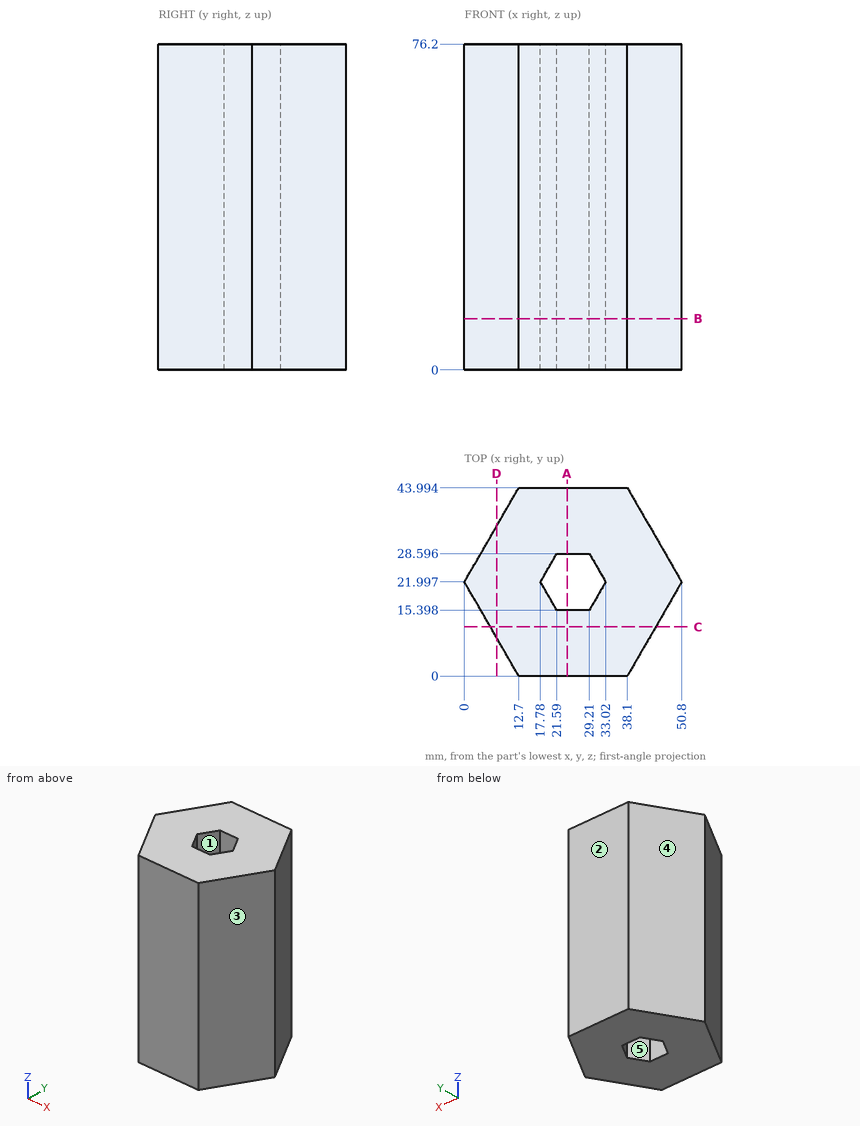
Part print with two shaded views. Sizes in mm from the minimum x, y, z corner. A direction names the side the tool comes from. Coordinates: 2 decimals unless noted, no trailing zeros. Loops run counter-clockwise (first coordinate to the right, second up) from the corner with the lowest first, then second, coordinate; pieces in that order, holes last. Notation, with made-up numbers: M -39.5,53.25 L 4.5,53.25 A7 cw 4.5,66.25 Z; hole C 53,39 d6. An arc over 180 degrees is marked long. Use CSV: the item, a comma, the result in double quotes. Start each with the question number.
1. Probe probe 1 along Y at (x, z) = (27, 12); probe 2 along Y at (x, z) = (47, 5) (1 decimal); probe 3 along Y at (x, z) = (32, 17). List the from-to ranges inside material, lowest first. Write a range as [from, to].
2. Two-plate mould, pull along Y, no slides. Class the marked faces 3, 4 and 5: pulls with the +Y half, pulls with the -Y half, needs draft (parallel to the pull), parting line crosses it, or undercut.
3. Band-saw the part on C-C, the plane y = 11.5. List the corners of the cut face in (x, z), then the cut area to 3 significant figures.
4. Band-saw the part on A-A, the plane x = 24. List the corners of the cut face in (y, z).
5. Tool access for the marked faces 1 and 2: list every direction of +Z, -Z, +X, -X, +Y, -Y with a clear straight run to the whole face (end or side of a thin tool).
6. Band-saw the part on D-D, the plane x = 7.5. List the corners of the cut face in (y, z).
7. Band-saw the part on B-B, the plane z = 12. List the corners of the cut face in (x, y).
8. Flat gauge pins, fed straight in: pin 1 (12 mm diameter, centred on x = 44.5, z = 62, fed in from -Y); pin 2 (12 mm diameter, centred on y = 34, z = 28.5, fed in from +X); pin 3 (12 mm diameter, centred on y = 8.5, z = 44.5, fed in from +X). Where does each tip first touch, or does it go through?
Entries:
1,probe 1,"y = [0, 15.4], [28.6, 43.99]"
1,probe 2,"y = [15.4, 28.6]"
1,probe 3,"y = [0, 20.23], [23.76, 43.99]"
2,face 3,"pulls with the -Y half"
2,face 4,"pulls with the +Y half"
2,face 5,"undercut"
3,outline,"M 6.06,0 L 44.74,0 L 44.74,76.2 L 6.06,76.2 Z"
3,area,"2,950 mm2"
4,outline,"M 0,0 L 15.4,0 L 15.4,76.2 L 0,76.2 Z; M 28.6,0 L 43.99,0 L 43.99,76.2 L 28.6,76.2 Z"
5,face 1,"+Z, -Z"
5,face 2,"+Z, -Z, +X, -X, +Y"
6,outline,"M 9.01,0 L 34.99,0 L 34.99,76.2 L 9.01,76.2 Z"
7,outline,"M 0,22 L 12.7,0 L 38.1,0 L 50.8,22 L 38.1,43.99 L 12.7,43.99 Z; hole M 17.78,22 L 21.59,15.4 L 29.21,15.4 L 33.02,22 L 29.21,28.6 L 21.59,28.6 Z"
8,pin 1,"stops at y = 0.69"
8,pin 2,"stops at x = 47.33"
8,pin 3,"stops at x = 46.47"
